Autodesk Inventor part; units mm, degrees
ref_plane "YZ Plane" through (0, 0, 0) normal (1, 0, 0) x (0, 1, 0)
ref_plane "XZ Plane" through (0, 0, 0) normal (0, 1, 0) x (-1, 0, 0)
ref_plane "XY Plane" through (0, 0, 0) normal (0, 0, 1) x (1, 0, 0)
sketch "Sketch1" plane through (0, 0, 0) normal (0, 0, 1) x (1, 0, 0)
  line L0 (11, 50) -> (-11, 50)
  line L1 (-15, 46) -> (-15, -46)
  line L2 (-11, -50) -> (-10, -50)
  line L3 (-6, -46) -> (-6, -45)
  line L4 (-6, -45) -> (-1, -10)
  line L5 (-1, -10) -> (-1, 0)
  line L6 (-1, 0) -> (4, 35)
  line L7 (4, 35) -> (4, 40)
  arc A0 (-10, -50) -> (-6, -46) centre (-10, -46) ccw
  arc A1 (-15, -46) -> (-11, -50) centre (-11, -46) ccw
  arc A2 (-11, 50) -> (-15, 46) centre (-11, 46) ccw
  line L8 (4, 40) -> (11, 40)
  line L9 (15, 44) -> (15, 46)
  arc A3 (15, 46) -> (11, 50) centre (11, 46) ccw
  arc A4 (11, 40) -> (15, 44) centre (11, 44) ccw
  point P0 (0, 0)
  point P1 (-15, 50)
  point P2 (-15, -50)
  point P3 (-6, -50)
  point P4 (-15, 0)
  point P5 (0, 50)
  dimension "d0" = 19
  dimension "d1" = 14
  dimension "d2" = 100
  dimension "d3" = 9
  dimension "d4" = 4
  dimension "d5" = 4
  dimension "d6" = 30
  dimension "d7" = 45
  dimension "d9" = 10
  dimension "d10" = 5
extrude "Extrusion1" add sketch "Sketch1" along normal blind 3
properties part number "Pin" material "Polycarbonate, Clear"
Geometry: final body of the model. Coordinates: model frame, mm. A direction names the side the tool comes from. Give positions to 0.01 mm unless a question says otherwise; leave off trailing zeros. Order: outer loops, then holes, each group sorted by start corner. A loop starts at its lowest first (then second) coordinate and runs counter-clockwise, first axis right, second up. Notation, with made-up numbers: M 86.25,55 L 101.25,55 A26 ccw 101.25,92 Z; hole C -21,36 d9. An arc over 180 degrees is marked long. Answer as CSV lines item,"result". Start each with the question number.
1) Cut plane B-B (y = -6.5). Output: boundary loops of the cut face in (x, z), then the cut area to 3 significant figures.
2) Set-up query: faces 1 (the flat face through (4, 37, 1)), 2 (the cylindrical face through (-13.859, 48.797, 1.479)). Return all of +Z, -Z, +X, -X, +Y, -Y with unobstructed straight access to the full face (end or side cutting, diameter ignored); none if empty.
3) Cut plane A-A (z = 1.55). Output: boundary loops of the cut face in (x, y).
4) Line query: line 1 (X direction, y = -8, z = 1.45); line 2 (X direction, y = -45.5, z = 1.7); line 3 (Y direction, x = 13, z = 2.6). Output: solid intervals per line, ascending. Write a range as from..to.
5) First-contact query: P1, Ø1.1, axis at y = -45.5, z = 1, coming from the +X side; P2, Ø0.9, axis at x = 9, z = 1.5, coming from the -Y side; P3, Ø12, axis at x = -9.5, y = -0.5, coming from the -Z side; P4, Ø0.9, axis at y = 37.5, z = 2, coming from the +X side. Flat tips, straight axial feed; report the tip coordinate or a pass-through.
6) Cut plane C-C (x = 2). Output: boundary loops of the cut face in (y, z).
Findings below:
1,outline,"M -15,0 L -1,0 L -1,3 L -15,3 Z"
1,area,"42.0 mm²"
2,face 1,"+Z, -Z, +X, -Y"
2,face 2,"+Z, -Z, -X, +Y"
3,outline,"M -15,-46 A4 ccw -11,-50 L -10,-50 A4 ccw -6,-46 L -6,-45 L -1,-10 L -1,0 L 4,35 L 4,40 L 11,40 A4 ccw 15,44 L 15,46 A4 ccw 11,50 L -11,50 A4 ccw -15,46 Z"
4,line 1,"x = -15..-1"
4,line 2,"x = -15..-6"
4,line 3,"y = 40.54..49.46"
5,P1,"stops at x = -5.99"
5,P2,"stops at y = 40"
5,P3,"stops at z = 0"
5,P4,"stops at x = 4"
6,outline,"M 21,0 L 50,0 L 50,3 L 21,3 Z"
